Autodesk Inventor part; units mm, degrees
ref_plane "YZ Plane" through (0, 0, 0) normal (1, 0, 0) x (0, 1, 0)
ref_plane "XZ Plane" through (0, 0, 0) normal (0, 1, 0) x (-1, 0, 0)
ref_plane "XY Plane" through (0, 0, 0) normal (0, 0, 1) x (1, 0, 0)
sketch "Sketch1" plane through (0, 0, 0) normal (0, 0, 1) x (1, 0, 0)
  line L0 (60, 0) -> (60, -27.025)
  line L1 (-60, -27.025) -> (-60, 0)
  line L2 (0, 54.7321) -> (0, -29.5526) construction
  line L3 (-1, -29.225) -> (-1, -27.025)
  line L4 (-1, -27.025) -> (1, -27.025)
  line L5 (1, -27.025) -> (1, -29.225)
  line L6 (-5, -29.225) -> (-5, -27.025)
  line L7 (-5, -27.025) -> (-3, -27.025)
  line L8 (-3, -27.025) -> (-3, -29.225)
  line L9 (3, -29.225) -> (3, -27.025)
  line L10 (3, -27.025) -> (5, -27.025)
  line L11 (5, -27.025) -> (5, -29.225)
  line L12 (-3, -29.225) -> (-1, -29.225)
  line L13 (1, -29.225) -> (3, -29.225)
  line L14 (-44.7, -29.225) -> (-44.7, -27.025)
  line L15 (-44.7, -27.025) -> (-46.7, -27.025)
  line L16 (-46.7, -27.025) -> (-46.7, -29.225)
  line L17 (-48.7, -29.225) -> (-48.7, -27.025)
  line L18 (-48.7, -27.025) -> (-50.7, -27.025)
  line L19 (-50.7, -27.025) -> (-50.7, -29.225)
  line L20 (-52.7, -29.225) -> (-50.7, -29.225)
  line L21 (-48.7, -29.225) -> (-46.7, -29.225)
  line L22 (-44.7, -29.225) -> (-5, -29.225)
  line L23 (44.7, -29.225) -> (44.7, -27.025)
  line L24 (44.7, -27.025) -> (46.7, -27.025)
  line L25 (46.7, -27.025) -> (46.7, -29.225)
  line L26 (48.7, -29.225) -> (48.7, -27.025)
  line L27 (48.7, -27.025) -> (50.7, -27.025)
  line L28 (50.7, -27.025) -> (50.7, -29.225)
  line L29 (5, -29.225) -> (44.7, -29.225)
  line L30 (46.7, -29.225) -> (48.7, -29.225)
  line L31 (50.7, -29.225) -> (52.7, -29.225)
  line L32 (-55.5, -31.525) -> (55.5, -31.525)
  line L33 (57.5, -21.825) -> (55.5, -21.825)
  line L34 (55.5, -21.825) -> (55.5, -19.825)
  line L35 (55.5, -19.825) -> (57.5, -19.825)
  line L36 (57.5, -17.825) -> (55.5, -17.825)
  line L37 (55.5, -17.825) -> (55.5, -15.825)
  line L38 (55.5, -15.825) -> (57.5, -15.825)
  line L39 (57.5, -24.225) -> (57.5, -21.825)
  line L40 (57.5, -19.825) -> (57.5, -17.825)
  line L41 (57.5, -15.825) -> (57.5, -8.1888)
  line L42 (57.5, -24.225) -> (54.9678, -24.225)
  line L43 (-57.5, -21.825) -> (-55.5, -21.825)
  line L44 (-55.5, -21.825) -> (-55.5, -19.825)
  line L45 (-55.5, -19.825) -> (-57.5, -19.825)
  line L46 (-57.5, -17.825) -> (-55.5, -17.825)
  line L47 (-55.5, -17.825) -> (-55.5, -15.825)
  line L48 (-55.5, -15.825) -> (-57.5, -15.825)
  line L49 (-57.5, -21.825) -> (-57.5, -24.225)
  line L50 (-57.5, -9.9008) -> (-57.5, -15.825)
  line L51 (-57.5, -17.825) -> (-57.5, -19.825)
  arc A0 (-60, -27.025) -> (-55.5, -31.525) centre (-55.5, -27.025) ccw
  arc A1 (55.5, -31.525) -> (60, -27.025) centre (55.5, -27.025) ccw
  arc A2 (54.0511, -26.6368) -> (55.1118, -25.5761) centre (55.5, -27.025) ccw
  arc A3 (-55.1118, -25.5761) -> (-54.0511, -26.6368) centre (-55.5, -27.025) ccw
  line L52 (52.7, -26.4928) -> (52.7, -29.225)
  line L53 (54.6142, -25.0786) -> (55.1118, -25.5761)
  line L54 (53.5536, -26.1392) -> (54.0511, -26.6368)
  line L55 (55.5, -27.025) -> (52.7, -24.225) construction
  arc A4 (54.9678, -24.225) -> (54.6142, -25.0786) centre (54.9678, -24.725) ccw
  arc A5 (53.5536, -26.1392) -> (52.7, -26.4928) centre (53.2, -26.4928) ccw
  line L56 (-57.5, -24.225) -> (-54.9678, -24.225)
  line L57 (-52.7, -26.4928) -> (-52.7, -29.225)
  line L58 (-55.5, -27.025) -> (-52.7, -24.225) construction
  line L59 (-55.1118, -25.5761) -> (-54.6142, -25.0786)
  line L60 (-54.0511, -26.6368) -> (-53.5536, -26.1392)
  arc A6 (-54.6142, -25.0786) -> (-54.9678, -24.225) centre (-54.9678, -24.725) ccw
  arc A7 (-52.7, -26.4928) -> (-53.5536, -26.1392) centre (-53.2, -26.4928) ccw
  line L61 (-57.5, -9.9008) -> (-55.5, -7.1508)
  line L62 (-55.5, -7.1508) -> (-55.5, 0)
  line L63 (57.5, -8.1888) -> (55.5, -4.7544)
  line L64 (55.5, -4.7544) -> (55.5, 0)
  arc A8 (-57, 1.3386) -> (-58.5, 1.3386) centre (-57.75, 2) ccw
  line L65 (-58.5, 0) -> (-58.5, 1.3386)
  line L66 (-57, 0) -> (-57, 1.3386)
  line L67 (-57.75, 1.7435) -> (-57.75, 0.7418) construction
  line L68 (-60, 0) -> (-58.5, 0)
  line L69 (-57, 0) -> (-55.5, 0)
  arc A9 (57, -1.3386) -> (58.5, -1.3386) centre (57.75, -2) ccw
  line L70 (57, -1.3386) -> (57, 0)
  line L71 (58.5, -1.3386) -> (58.5, 0)
  line L72 (57.75, 2.8392) -> (57.75, 0.4457) construction
  line L73 (55.5, 0) -> (57, 0)
  line L74 (58.5, 0) -> (60, 0)
  point P0 (0, 0)
  dimension "d0" = 120
  dimension "d11" = 2
  dimension "d13" = 39.7
  dimension "d14" = 2.3
  dimension "d16" = 4.5
  dimension "d17" = 10
  dimension "d19" = 7.3
  dimension "d20" = 8.4
  dimension "d21" = 115
  dimension "d22" = 111
  dimension "d23" = 9
  dimension "d25" = 3
  dimension "d26" = 7.3
  dimension "d28" = 1.5
  dimension "d29" = 1
  dimension "d31" = 1.5
  dimension "d32" = 2
  dimension "d34" = 1.5
  dimension "d35" = 31.525
  dimension "d36" = 2
  dimension "d37" = 1.5
  dimension "d38" = 2
  dimension "d41" = 111
extrude "Extrusion1" add sketch "Sketch1" along normal blind 20
equation "\"d26\" = d19"
equation "\"d31\" = d28"
equation "\"d36\" = d32"
equation "\"d37\" = d34"
properties part number "SZOMK-AK-C-C10"
The listing builds one solid part. Answer for the finished solid, in the listing's coordinates (mm). A direction names the side the tool comes from. Give positions to 0.01 mm unless a question says otherwise; leave off trailing zeros. Order: outer loops, then holes, each group sorted by start corner. A loop starts at its lowest first (then second) coordinate and runs counter-clockwise, first axis right, second up. Notation, with made-up numbers: (-19.5, 16) - (-5.5, 16) arc R24 ccw to (-5.5, 48) - close; hole circle Ø7 at (15.5, 10.5). An arc over 180 degrees is marked (long way). Answer in a Markdown table with one row per item. Add a question column.
Q1. Find the intervals of material crossed by line 1 along X through (y, z) = (-2, 11.25); line 2 along X through (y, z) = (-23, 11); line 3 along X through (y, z) = (-1, 14.5), in increasing order. Write a range as [from, to].
Q2. Given P1, Ø3, axis at x = 13, z = 7, coming from the +Y side (3 decimals); P2, Ø0.8, axis at x = 59, z = 6, coming from the +Y side; P3, Ø1, axis at x = -4.5, z = 13.5, coming from the +Y side (3 decimals), each flat-ended and moving along its own axis, determine where each tip first touches the part or whether it passes through.
Q3. Which of the six approach directions +Z, -Z, +X, -X, +Y, -Y give full straight-line access (tool end or side, diameter ignored) to faces 1 (the flat face through (57, -17.825, 10)), 2 (the flat face through (48.7, -28, 10)), 3 (the flat face through (60, -13, 10))?
Q4. The part is cut by section A-A (x = -33). Determine the outline of the cut face in (y, z) (3 decimals).
Determined:
| question | item | result |
|---|---|---|
| 1 | line 1 | x = [-60, -55.5], [55.5, 56.75], [58.75, 60] |
| 1 | line 2 | x = [-60, -57.5], [57.5, 60] |
| 1 | line 3 | x = [-60, -55.5], [55.5, 57], [58.5, 60] |
| 2 | P1 | stops at y = -29.225 |
| 2 | P2 | stops at y = 0 |
| 2 | P3 | stops at y = -27.025 |
| 3 | face 1 | +Z, -Z |
| 3 | face 2 | +Z, -Z, +Y |
| 3 | face 3 | +Z, -Z, +X, +Y, -Y |
| 4 | outline | (-31.525, 0) - (-29.225, 0) - (-29.225, 20) - (-31.525, 20) - close |
